from build123d import *

# Parameters (mm, degrees)
SKETCH1_W           = 4.5
SKETCH1_H           = 4.5
BOSS_EXTRUDE3_DEPTH = 1


with BuildPart() as part:
    # Sketch1 → Boss-Extrude3 (new body)
    with BuildSketch(Plane(origin=(0, 0, 0), x_dir=(1, 0, 0), z_dir=(0, 1, 0))):
        Polygon((122.038308787, 26.301002263), (52.538308787, 26.301002263), (52.538308787, -8.448997737), (51.538308787, -8.448997737), (51.538308787, 26.301002263), (-17.961691213, 26.301002263), (-17.961691213, -43.198997737), (16.788308787, -43.198997737), (16.788308787, -44.198997737), (-17.961691213, -44.198997737), (-17.961691213, -113.698997737), align=None)
        with Locations((-2.961691213, 11.301002263)):
            Rectangle(SKETCH1_W, SKETCH1_H, mode=Mode.SUBTRACT)
        with Locations((107.038308787, 18.801002263)):
            Rectangle(SKETCH1_W, SKETCH1_H, mode=Mode.SUBTRACT)
        with Locations((-10.461691213, -98.698997737)):
            Rectangle(SKETCH1_W, SKETCH1_H, mode=Mode.SUBTRACT)
    extrude(amount=BOSS_EXTRUDE3_DEPTH)


solid = part.part
The model under review builds one solid part; all positions refer to its coordinate system, in mm. Give positions to 0.01 mm unless a question says otherwise; leave off trailing zeros. Write each loop counter-clockwise with the first axis right and the second up, starting at its lowest first coordinate (ties: lowest second). Pieces come first, ordered by that corner, then holes. Notation, with made-up numbers: M -21,-34.75 L -2,-34.75 A20 ccw -2,-3.75 Z; hole C 12,-31.75 d3. An arc over 180 degrees is marked long. One line per question, with ' | ' between items. Start each with the question number.
Item 1: We need section A-A on y = 0.15. Write out the cut boundary in (x, z), plus the area to 3 significant figures.
Item 2: We need section C-C on z = -2. Write out the cut boundary in (x, y), plus the area to 3 significant figures.
Item 3: Wall thickness on line 1 (Z direction, x = 107, y = 0.3); line 2 (X direction, y = 0.35, z = 98.5); line 3 (X direction, y = 0.5, z = 6): over which ranges is each line inside the solid? List them lowest first. Write a range as from..to.
Item 4: We need section B-B on x = 6. Write out the cut boundary in (y, z), plus the area to 3 significant figures.
Item 5: We need section D-D on x = 38. Write out the cut boundary in (y, z).
Item 6: For pin 1 (0.5 mm diameter, centred on y = 0.5, z = -18.5, fed in from +X); pin 2 (0.5 mm diameter, centred on x = -3, y = 0.5, fed in from +Z), all flat-tipped, find the tip position at first contact; note any pin that passes through.
Results found:
1) outline: M -17.96,-26.3 L 51.54,-26.3 L 51.54,8.45 L 52.54,8.45 L 52.54,-26.3 L 122.04,-26.3 L -17.96,113.7 L -17.96,44.2 L 16.79,44.2 L 16.79,43.2 L -17.96,43.2 Z; hole M -12.71,96.45 L -8.21,96.45 L -8.21,100.95 L -12.71,100.95 Z; hole M -5.21,-13.55 L -0.71,-13.55 L -0.71,-9.05 L -5.21,-9.05 Z; hole M 104.79,-21.05 L 109.29,-21.05 L 109.29,-16.55 L 104.79,-16.55 Z | area: 9,670 mm2
2) outline: M -17.96,0 L 51.54,0 L 51.54,1 L -17.96,1 Z; M 52.54,0 L 97.74,0 L 97.74,1 L 52.54,1 Z | area: 115 mm2
3) line 1: z = -26.3..-21.05, -16.55..-11.26 | line 2: x = -17.96..-12.71, -8.21..-2.76 | line 3: x = -17.96..51.54, 52.54..89.74
4) outline: M 0,-26.3 L 1,-26.3 L 1,43.2 L 0,43.2 Z; M 0,44.2 L 1,44.2 L 1,89.74 L 0,89.74 Z | area: 115 mm2
5) outline: M 0,-26.3 L 1,-26.3 L 1,57.74 L 0,57.74 Z
6) pin 1: stops at x = 114.49 | pin 2: stops at z = 98.99
